```python
from build123d import *

# Parameters (mm, degrees)
F0_W     = 66.0715028644
F0_H     = 81.7836225033
F1_DEPTH = 32.004
F2_R     = 19.6431744844
F3_DEPTH = 63.246
F4_R     = 25.3969139416
F4_R_2   = 19.6431744844
F5_DEPTH = 25.4


with BuildPart() as f1:
    # F0 (on Top) → F1 (new body)
    with BuildSketch(Plane.XY):
        with Locations((0.6206892431, -1.0830126703)):
            Rectangle(F0_W, F0_H)
    extrude(amount=F1_DEPTH)

    # F2 (on face) → F3 (cut)
    with BuildSketch(Plane.XY.offset(32.004)):
        Circle(F2_R)
    extrude(amount=-F3_DEPTH, mode=Mode.SUBTRACT)

    # F4 (on face) → F5 (join)
    with BuildSketch(Plane.XY.offset(32.004)):
        Circle(F4_R)
        Circle(F4_R_2, mode=Mode.SUBTRACT)
    extrude(amount=F5_DEPTH)


solid = f1.part
```
Work out the finished part from the listing and answer in its coordinate system (mm). A direction names the side the tool comes from. Give positions to 0.01 mm unless a question says otherwise; leave off trailing zeros. Loops run counter-clockwise (first coordinate to the right, second up) from the corner with the lowest first, then second, coordinate; pieces in that order, holes last. Notation, with made-up numbers: M 3,16.25 L 17,16.25 A32 cw 17,52.25 Z; hole C -1,-7.75 d4. An arc over 180 degrees is marked long. One line per item, written item: value. Start each with the question number.
1. Find section A-A (y = 0). Give the vertices of the cut face in (x, z), and give its area (3 significant figures).
2. Find the intervals of material crossed by probe 1 along Y at (x, z) = (0, 22.5); probe 2 along Y at (x, z) = (0, 49); probe 3 along Z at (x, y) = (18, -32), in increasing order.
3. Each of these flat-tipped pins is pushed along its axis until it touches: P1, Ø8, axis at x = 6.5, z = 37, coming from the -Y side; P2, Ø4, axis at x = 23, z = 35, coming from the -Y side; P3, Ø2, axis at y = 6, z = 42, coming from the +X side. Where does it stop, or does it pass through?
4. Find section D-D (x = -23). Give the vertices of the cut face in (y, z), and give its area (3 significant figures).
5. Find section B-B (x = 0). Give the vertices of the cut face in (y, z).
6. Find section C-C (z = 21). Give the vertices of the cut face in (x, y).
7. Which of the six approach directions +Z, -Z, +X, -X, +Y, -Y give full straight-line access (tool end or side, diameter ignored) to faces 1 (the face through (0, -41.975, 16)), 2 (the face through (0, 27, 32.004))?
Reported:
1. outline: M -32.42,0 L -19.64,0 L -19.64,57.4 L -25.4,57.4 L -25.4,32 L -32.42,32 Z; M 19.64,0 L 33.66,0 L 33.66,32 L 25.4,32 L 25.4,57.4 L 19.64,57.4 Z
1. area: 1,150 mm²
2. probe 1: y = -41.97 to -19.64, 19.64 to 39.81
2. probe 2: y = -25.4 to -19.64, 19.64 to 25.4
2. probe 3: z = 0 to 32
3. P1: stops at y = -25.27
3. P2: stops at y = -14.28
3. P3: stops at x = 24.9
4. outline: M -41.97,0 L 39.81,0 L 39.81,32 L 10.77,32 L 10.77,57.4 L -10.77,57.4 L -10.77,32 L -41.97,32 Z
4. area: 3,160 mm²
5. outline: M -41.97,0 L -19.64,0 L -19.64,57.4 L -25.4,57.4 L -25.4,32 L -41.97,32 Z; M 19.64,0 L 39.81,0 L 39.81,32 L 25.4,32 L 25.4,57.4 L 19.64,57.4 Z
6. outline: M -32.42,-41.97 L 33.66,-41.97 L 33.66,39.81 L -32.42,39.81 Z; hole C 0,0 d39.29
7. face 1: +Z, -Z, +X, -X, -Y
7. face 2: +Z
